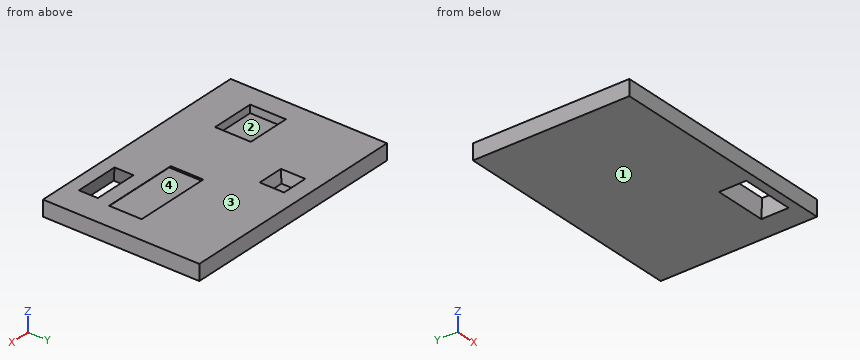
from build123d import *

# Parameters (mm, degrees)
F0_W      = 300
F0_H      = 200
F1_DEPTH  = 20
F2_W      = 56.0527034104
F2_H      = 45.7135215402
F3_DEPTH  = 10
F4_W      = 66.9058933854
F4_H      = 34.0227484703
F5_DEPTH  = 10
F6_W      = 98.600897938
F6_H      = 41.7043203488
F7_DEPTH  = 10
F7_TAPER  = -45
F8_W      = 32.641120255
F8_H      = 31.1660170555
F9_DEPTH  = 10
F9_TAPER  = -20
F10_W     = 33.9855737984
F10_H     = 31.0657545924
F11_DEPTH = 15
F11_TAPER = 10
F12_W     = 56.9754764438
F12_H     = 24.2112912238
F13_DEPTH = 25
F13_TAPER = -15


with BuildPart() as f1:
    # F0 (on Top) → F1 (new body)
    with BuildSketch(Plane.XY):
        with Locations((19.8950484647, 29.7908782959)):
            Rectangle(F0_W, F0_H)
    extrude(amount=F1_DEPTH)

    # F2 (on face) → F3 (cut)
    with BuildSketch(Plane.XY.offset(20)):
        with Locations((-75.3318350762, -1.0474342853)):
            Rectangle(F2_W, F2_H)
    extrude(amount=-F3_DEPTH, mode=Mode.SUBTRACT)

    # F4 (on face) → F5 (join)
    with BuildSketch(Plane.XY.offset(20)):
        with Locations((92.6642976701, 79.7481462359)):
            Rectangle(F4_W, F4_H)
    extrude(amount=-F5_DEPTH)

    # F6 (on face) → F7 (cut)
    with BuildSketch(Plane.XY.offset(20)):
        with Locations((88.7664388865, 9.6967569552)):
            Rectangle(F6_W, F6_H)
    extrude(amount=-F7_DEPTH, taper=F7_TAPER, mode=Mode.SUBTRACT)

    # F8 (on face) → F9 (join)
    with BuildSketch(Plane.XY.offset(20)):
        with Locations((-97.8116877377, 101.3978421688)):
            Rectangle(F8_W, F8_H)
    extrude(amount=-F9_DEPTH, taper=F9_TAPER)

    # F10 (on face) → F11 (cut)
    with BuildSketch(Plane.XY.offset(20)):
        with Locations((-8.2211010158, 93.6475135386)):
            Rectangle(F10_W, F10_H)
    extrude(amount=-F11_DEPTH, taper=F11_TAPER, mode=Mode.SUBTRACT)

    # F12 (on face) → F13 (cut)
    with BuildSketch(Plane.XY.offset(20)):
        with Locations((104.9904711545, -41.3090791553)):
            Rectangle(F12_W, F12_H)
    extrude(amount=-F13_DEPTH, taper=F13_TAPER, mode=Mode.SUBTRACT)


solid = f1.part
Design review of the part built by this model. Coordinates are the model's own, in mm. Face numbers are marked on the shaded views. A direction names the side the tool comes from. Coordinates: 2 decimals unless noted, no trailing zeros. Write each loop counter-clockwise with the first axis right and the second up, starting at its lowest first coordinate (ties: lowest second). Pieces come first, ordered by that corner, then holes. Notation, with made-up numbers: (-30.5, 38) - (-12.5, 38) arc R19 cw to (-12.5, 69) - close; hole circle Ø10 at (24, 40.25). An arc over 180 degrees is marked (long way). Use one line per item in the form item = value.
Q1. For probe 1 along Y at (x, z) = (-96, 14.75); probe 2 along Y at (x, z) = (87, 12.5); probe 3 along Y at (x, z) = (130.5, 16), list the stretches that pass through material, from the lowest coordinate up.
Taken from the geometry:
probe_1 = -70.21 to -23.9, 21.81 to 129.79
probe_2 = -70.21 to -55.42, -27.19 to -18.66, 38.05 to 129.79
probe_3 = -70.21 to -54.49, -28.13 to -15.16, 34.55 to 129.79
Q2. Consider section A-A (x = -65). Write out the cut boundary in (y, z), plus the area to 3 significant figures.
Taken from the geometry:
outline = (-70.21, 0) - (129.79, 0) - (129.79, 20) - (21.81, 20) - (21.81, 10) - (-23.9, 10) - (-23.9, 20) - (-70.21, 20) - close
area = 3,540 mm^2
Q3. Consider section B-B (z = 14). Count the separate pieces of the cut face and the enclosed holes in it, plus the area to 3 significant figures.
Taken from the geometry:
separate_pieces = 1
enclosed_holes = 4
area = 48,900 mm^2
Q4. Machinability: for the marked faces 3 and 4, which of the approach directions +Z, -Z, +X, -X, +Y, -Y give a long, thin tool a straight path to every point of the face, cutting with its end or side? Answer none if there is none.
Taken from the geometry:
face_3 = +Z, +X, -X, +Y, -Y
face_4 = none
Q5. The part is to be moulded in two halves that separate along Y. For the marked faces 1 and 2, say which applies: +Y half, -Y half, draft (parallel to the pull), parting line (faces both ways), or undercut.
Taken from the geometry:
face_1 = draft
face_2 = undercut
